Here's how the part is built. I have some questions about the finished solid (model axes, mm). A direction names the side the tool comes from. Round coordinates to 2 decimals unless told otherwise and drop trailing zeros. Order: outer loops, then holes, each group sorted by start corner. A loop starts at its lowest first (then second) coordinate and runs counter-clockwise, first axis right, second up. Notation, with made-up numbers: (2.25, -12) -> (25.25, -12) arc R5 cw to (25.25, -8) -> close; hole circle Ø7 at (12, -16). An arc over 180 degrees is marked (long way). One line per item, written item: value.
```python
from build123d import *

# Parameters (mm, degrees)
EXTRUDE_1_DEPTH     = 10
SKETCH_2_R          = 5
CUT_EXTRUDE_1_DEPTH = 10
SKETCH_3_W          = 250
SKETCH_3_H          = 250
EXTRUDE_2_DEPTH     = 125
SKETCH_5_W          = 250
SKETCH_5_H          = 250
CUT_EXTRUDE_2_DEPTH = 95
SKETCH_8_W          = 250
SKETCH_8_H          = 250
SKETCH_8_W_2        = 153.371517144
SKETCH_8_H_2        = 151.494592983
CUT_EXTRUDE_4_DEPTH = 10
CUT_EXTRUDE_5_DEPTH = 352.385042723
SKETCH_10_R         = 5
CUT_EXTRUDE_7_DEPTH = 287.71149486
SKETCH_12_R         = 5
CUT_EXTRUDE_8_DEPTH = 287.71149486


with BuildPart() as part:
    # 草图1 → 凸台-拉伸1 (new body)
    with BuildSketch(Plane.XY):
        with BuildLine():
            Line((-217.911131847, 17.366483315), (-57.911131847, 17.366483315))
            ThreePointArc((-57.911131847, 17.366483315), (-47.911131847, 7.366483315), (-57.911131847, -2.633516685))
            Line((-57.911131847, -2.633516685), (-217.911131847, -2.633516685))
            Line((-217.911131847, -2.633516685), (-217.911131847, 17.366483315))
        make_face()
    extrude(amount=EXTRUDE_1_DEPTH)

    # 草图2 → 切除-拉伸1 (cut)
    with BuildSketch(Plane.XY.offset(10)):
        with Locations((-57.911131847, 7.366483315)):
            Circle(SKETCH_2_R)
        with Locations((-7.911347857, 7.219510907)):
            Circle(SKETCH_2_R)
    extrude(amount=-CUT_EXTRUDE_1_DEPTH, mode=Mode.SUBTRACT)

    # 草图3 → 凸台-拉伸2 (add)
    with BuildSketch(Plane.XZ.offset(2.633516685)):
        with Locations((-198.652892484, 10.352330738)):
            Rectangle(SKETCH_3_W, SKETCH_3_H)
    extrude(amount=-EXTRUDE_2_DEPTH)

    # 草图4 → 切除-旋转1 (revolve, cut)
    with BuildSketch(Plane(origin=(0, 122.366483315, 0), x_dir=(1, 0, 0), z_dir=(0, 1, 0))):
        with BuildLine():
            Line((-283.505706227, 74.500483004), (-113.800078742, -95.205144481))
            ThreePointArc((-113.800078742, -95.205144481), (-283.505706227, -95.205144481), (-283.505706227, 74.500483004))
        make_face()
    revolve(axis=Axis((-283.505706227, 122.366483315, -74.500483004), (0.7071067811865477, 0, 0.7071067811865474)), mode=Mode.SUBTRACT)

    # 草图5 → 切除-拉伸2 (cut)
    with BuildSketch(Plane(origin=(0, 122.366483315, 0), x_dir=(1, 0, 0), z_dir=(0, 1, 0))):
        with Locations((-198.652892484, -10.352330738)):
            Rectangle(SKETCH_5_W, SKETCH_5_H)
    extrude(amount=-CUT_EXTRUDE_2_DEPTH, mode=Mode.SUBTRACT)

    # 草图8 → 切除-拉伸4 (cut)
    with BuildSketch(Plane(origin=(0, 27.366483315, 0), x_dir=(1, 0, 0), z_dir=(0, 1, 0))):
        with Locations((-198.652892484, -10.352330738)):
            Rectangle(SKETCH_8_W, SKETCH_8_H)
        with Locations((-198.384057314, -10.352330739)):
            Rectangle(SKETCH_8_W_2, SKETCH_8_H_2, mode=Mode.SUBTRACT)
    extrude(amount=-CUT_EXTRUDE_4_DEPTH, mode=Mode.SUBTRACT)

    # 草图9 → 切除-拉伸5 (cut, through all)
    with BuildSketch(Plane(origin=(0, 17.366483315, 0), x_dir=(1, 0, 0), z_dir=(0, 1, 0))):
        Polygon((-275.069815886, -86.09962723), (-275.069815886, 65.394965753), (-121.698298742, 65.394965753), (-121.698298742, 0), (-73.652892484, 0), (-73.652892484, 114.647669262), (-323.652892484, 114.647669262), (-323.652892484, -135.352330738), (-73.652892484, -135.352330738), (-73.652892484, -10), (-121.698298742, -10.352330738), (-121.698298742, -86.09962723), align=None)
    extrude(amount=-CUT_EXTRUDE_5_DEPTH, mode=Mode.SUBTRACT)

    # 草图10 → 切除-拉伸7 (cut, through all)
    with BuildSketch(Plane.XY.offset(10)):
        with Locations((-107.91077949, 7.55419482)):
            Circle(SKETCH_10_R)
    extrude(amount=-CUT_EXTRUDE_7_DEPTH, mode=Mode.SUBTRACT)

    # 草图12 → 切除-拉伸8 (cut, through all)
    with BuildSketch(Plane(origin=(0, 0, 10), x_dir=(-1, 0, 0), z_dir=(0, 0, -1))):
        with Locations(Location((107.91077949, 7.55419482, 0), (0, 0, 180))):
            Circle(SKETCH_12_R)
    extrude(amount=-CUT_EXTRUDE_8_DEPTH, mode=Mode.SUBTRACT)


solid = part.part
```
Q1. I want a section at C-C on y = 23. Write out the boundary of the cut face in (x, z).
Answers:
outline: (-275.07, -65.39) -> (-121.7, -65.39) -> (-121.7, 86.1) -> (-275.07, 86.1) -> close; hole circle Ø134.56 at (-198.65, 10.35)
Q2. I want a section at B-B on z = 17. Write out the boundary of the cut face in (x, y), then the cut area to 3 significant figures.
Answers:
outline: (-275.07, -2.63) -> (-121.7, -2.63) -> (-121.7, 27.37) -> (-125.64, 27.37) arc R119.82 cw to (-271.67, 27.37) -> (-275.07, 27.37) -> close
area: 2,130 mm2
Q3. I need wall thicknesses on line 1 along X through (y, z) = (12, -37); line 2 along Z through (x, y) = (-233, 21.5); line 3 along Z through (x, y) = (-178.5, 24.25). Which ranges of each line are inside material? Lowest first, please.
Answers:
line 1: -275.07 to -121.7
line 2: -65.39 to -44.84, 65.54 to 86.1
line 3: -65.39 to -55.73, 76.44 to 86.1
Q4. Which directions (+Z, -Z, +X, -X, +Y, -Y) give clear straight access to the entire face, cutting with the end or side of a thin tool? Please do faces 1 (the face through (-63.5, 7.5, 10)), 2 (the face through (-90, 17.366, 5)), 3 (the face through (-197, 13, 86.1)).
Answers:
face 1: +Z, +X, +Y, -Y
face 2: +Z, -Z, +X, +Y
face 3: +Z, +X, -X, +Y, -Y
Q5. I want a section at D-D on x = -183.5. Write out the boundary of the cut face in (y, z).
Answers:
outline: (-2.63, -65.39) -> (27.37, -65.39) -> (27.37, -61.38) arc R119.04 cw to (27.37, 82.08) -> (27.37, 86.1) -> (-2.63, 86.1) -> close
Q6. I want a section at A-A on x = -66. Write out the boundary of the cut face in (y, z), then the cut area to 3 significant figures.
Answers:
outline: (-2.63, 0) -> (17.37, 0) -> (17.37, 10) -> (-2.63, 10) -> close
area: 200 mm2
Q7. If we mould it in two halves opening along X, with no side actions, what happens to faces 4 (the face through (-275.07, 13, 11)), 5 (the face through (-85, 8, 0)), 6 (the face through (-47.914, 7.586, 4.93)), 7 (the face through (-62.906, 7.586, 5.07))? For each: pulls with the +X half, pulls with the -X half, needs draft (parallel to the pull), parting line crosses it, or undercut.
Answers:
face 4: pulls with the -X half
face 5: needs draft
face 6: pulls with the +X half
face 7: undercut
Q8. For P1, Ø11.5, axis at x = -57.91, y = 7.37, coming from the +Z side; P2, Ø6, axis at y = 24, z = 57, coming from the +X side; P3, Ø11.5, axis at x = -80.5, z = 6.5, coming from the +Y side, each with a flat end and sliding along its axis, tell me the tip position at first contact or that it passes through.
Answers:
P1: z = 10
P2: x = -121.7
P3: y = 17.37
